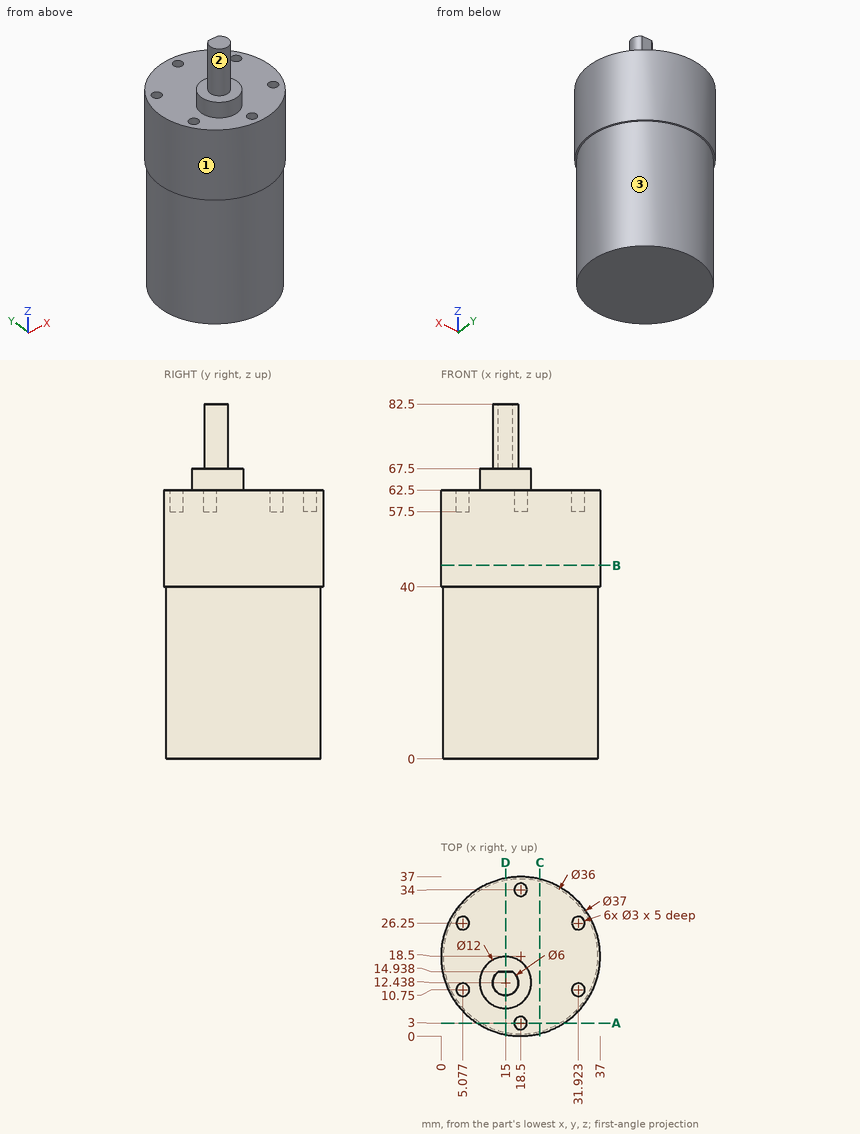
Design review of the part shown in the three views and the two pictorial views. Dimensions are in mm from the part's minimum x, y and z. A direction names the side the tool comes from. Give positions to 0.01 mm unless a question says otherwise; leave off trailing zeros. Loops run counter-clockwise (first coordinate to the right, second up) from the corner with the lowest first, then second, coordinate; pieces in that order, holes last. Notation, with made-up numbers: (-30.5, 22) -> (-5.5, 22) arc R28 cw to (-5.5, 47) -> close; hole circle Ø3 at (26.25, 61). An arc over 180 degrees is marked (long way). Write each question's results on one line, items separated by ' | '.
Q1. For pin 1 Ø2.5 at (x, y) = (31.92, 26.25) entering from +Z; pin 2 Ø2 at (x, z) = (27, 27.5) entering from +Y; pin 3 Ø2.5 at (x, y) = (18, 34) entering from +Z, all flat-tipped, find the tip position at first contact; note any pin that passes through.
Reply:
pin 1: stops at z = 57.5 | pin 2: stops at y = 34.86 | pin 3: stops at z = 62.5
Q2. Take a section at D-D, the plane x = 15. Write out the cut boundary in (y, z), plus the area to 3 significant figures.
Reply:
outline: (0.33, 40) -> (0.84, 40) -> (0.84, 0) -> (36.16, 0) -> (36.16, 40) -> (36.67, 40) -> (36.67, 62.5) -> (18.44, 62.5) -> (18.44, 67.5) -> (14.94, 67.5) -> (14.94, 82.5) -> (9.44, 82.5) -> (9.44, 67.5) -> (6.44, 67.5) -> (6.44, 62.5) -> (0.33, 62.5) -> close | area: 2,370 mm²
Q3. Take a section at B-B, the plane z = 45. Write out the cut boundary in (x, y).
Reply:
outline: circle Ø37 at (18.5, 18.5)
Q4. Wall thickness on L1, parallel to Y at x = 18.5, z = 61.1; L2, parallel to Z at x = 10, y = 25.5; L3, parallel to Y at x = 19, z = 21: over which ranges is each line inside the solid? List them lowest first.
Reply:
L1: y = 0 to 1.5, 4.5 to 32.5, 35.5 to 37 | L2: z = 0 to 62.5 | L3: y = 0.51 to 36.49
Q5. Take a section at A-A, the plane y = 3. Write out the cut boundary in (x, z).
Reply:
outline: (8.4, 40) -> (9.35, 40) -> (9.35, 0) -> (27.65, 0) -> (27.65, 40) -> (28.6, 40) -> (28.6, 62.5) -> (20, 62.5) -> (20, 57.5) -> (17, 57.5) -> (17, 62.5) -> (8.4, 62.5) -> close
Q6. Machinability: for the marked faces 1, 2 and 3, which of the approach directions +Z, -Z, +X, -X, +Y, -Y give a long, thin tool a straight path to every point of the face, cutting with its end or side? Answer none if there is none.
Reply:
face 1: +Z, -Z | face 2: +Z | face 3: -Z
Q7. Take a section at C-C, the plane x = 23. Write out the cut boundary in (y, z) (1 decimal).
Reply:
outline: (0.6, 40) -> (1.1, 40) -> (1.1, 0) -> (35.9, 0) -> (35.9, 40) -> (36.4, 40) -> (36.4, 62.5) -> (0.6, 62.5) -> close
